```python
from build123d import *

# Parameters (mm, degrees)
F0_W     = 114
F0_H     = 114
F1_DEPTH = 50
F2_T     = -3
F4_DEPTH = 114.001
F6_DEPTH = 114.001
F7_R     = 5
F8_R     = 2
F9_R     = 2


with BuildPart() as f1:
    # F0 (on Top) → F1 (new body)
    with BuildSketch(Plane.XY):
        with Locations((24.0205488801, 21.5819291472)):
            Rectangle(F0_W, F0_H)
    extrude(amount=F1_DEPTH)

    # F2
    f2_openings = [f1.faces().sort_by_distance(p)[0] for p in [
        (24.020549, 21.581929, 50),
    ]]
    offset(amount=F2_T, openings=f2_openings)

    # F3 (on face) → F4 (cut, through all)
    with BuildSketch(Plane(origin=(-32.9794511199, 0, 0), x_dir=(0, -1, 0), z_dir=(-1, 0, 0))):
        with BuildLine():
            Line((-12.5819291472, 19), (-12.5819291472, 50))
            Line((-12.5819291472, 50), (-30.5819291472, 50))
            Line((-30.5819291472, 50), (-30.5819291472, 19))
            ThreePointArc((-30.5819291472, 19), (-21.5819291472, 10), (-12.5819291472, 19))
        make_face()
    extrude(amount=-F4_DEPTH, mode=Mode.SUBTRACT)

    # F5 (on face) → F6 (cut, through all)
    with BuildSketch(Plane(origin=(0, 78.5819291472, 0), x_dir=(-1, 0, 0), z_dir=(0, 1, 0))):
        with BuildLine():
            Line((-33.0205488801, 50), (-33.0205488801, 19))
            ThreePointArc((-33.0205488801, 19), (-24.0205488801, 10), (-15.0205488801, 19))
            Line((-15.0205488801, 19), (-15.0205488801, 50))
            Line((-15.0205488801, 50), (-33.0205488801, 50))
        make_face()
    extrude(amount=-F6_DEPTH, mode=Mode.SUBTRACT)

    # F7
    f7_edges = [f1.edges().sort_by_distance(p)[0] for p in [
        (15.020549, 77.081929, 50),
        (15.020549, -33.918071, 50),
        (33.020549, 77.081929, 50),
        (33.020549, -33.918071, 50),
        (79.520549, 12.581929, 50),
        (-31.479451, 12.581929, 50),
        (79.520549, 30.581929, 50),
        (-31.479451, 30.581929, 50),
    ]]
    fillet(f7_edges, radius=F7_R)

    # F8
    f8_edges = [f1.edges().sort_by_distance(p)[0] for p in [
        (81.020549, -35.418071, 25),
        (-32.979451, -35.418071, 25),
        (-32.979451, 78.581929, 25),
        (81.020549, 78.581929, 25),
    ]]
    fillet(f8_edges, radius=F8_R)

    # F9
    f9_edges = [f1.edges().sort_by_distance(p)[0] for p in [
        (-29.979451, -32.418071, 26.5),
        (-29.979451, 75.581929, 26.5),
        (78.020549, 75.581929, 26.5),
        (78.020549, -32.418071, 26.5),
    ]]
    fillet(f9_edges, radius=F9_R)


solid = f1.part
```
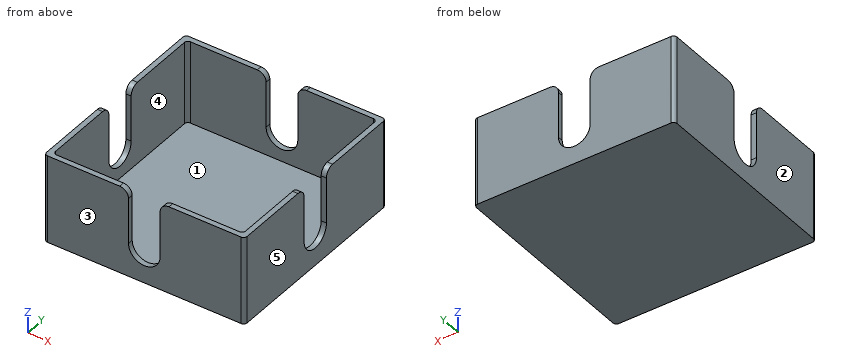
Geometry check sheet. Reference: the model listing, model coordinates, mm. Face numbers are marked on the shaded views. A direction names the side the tool comes from. Give positions to 0.01 mm unless a question says otherwise; leave off trailing zeros. Order: outer loops, then holes, each group sorted by start corner. A loop starts at its lowest first (then second) coordinate and runs counter-clockwise, first axis right, second up. Notation, with made-up numbers: (17.25, -21) - (32.25, -21) arc R16 cw to (32.25, -13) - close; hole circle Ø11 at (41.25, 68.5). An arc over 180 degrees is marked (long way). Answer in a Markdown table with one row per item. Add a question column.
Q1. Gauge pin test, flat ends, axial feed: pin 1 (8 mm diameter, centred on y = 20.5, z = 36.5, fed in from +X); pin 2 (2.5 mm diameter, centred on y = 77, z = 34.5, fed in from -X); pin 3 (4 mm diameter, centred on x = 69, y = 43, fed in from +Z). Record the tip position at first contact, or that the pin passes through.
Q2. Cross-section at C-C, the plane x = 63.5. Enter the section's corners in (y, z).
Q3. Material ranges on probe 1 along X at (y, z) = (-22, 3.5); probe 2 along Y at (x, z) = (-23, 19.5); probe 3 along Z at (x, y) = (7, 21.5), recorded low to high. Write a range as from..to.
Q4. Cross-section at B-B, the plane y = 40. Enter the section's corners in (x, z), then the cut area to 3 significant figures.
Q5. Tool access check on the marked faces 1 and 2. Record the directions out of +Z, -Z, +X, -X, +Y, -Y that give a thin tool (end or side, any length) a straight path to the whole face; none if there is none.
Q6. Cross-section at A-A, the plane z = 42. Count the separate pieces of the cut face and the enclosed holes in it, then the cut area to 3 significant figures.
Q7. Mould release check, pull along Y, two halves, no side actions. Record for the marked faces 3, 4 and 5: pulls with the +Y half, pulls with the -Y half, needs draft (parallel to the pull), parting line crosses it, or undercut.
Check values:
| question | item | result |
|---|---|---|
| 1 | pin 1 | passes through |
| 1 | pin 2 | stops at x = -32.98 |
| 1 | pin 3 | stops at z = 3 |
| 2 | outline | (-35.42, 0) - (78.58, 0) - (78.58, 50) - (75.58, 50) - (75.58, 3) - (-32.42, 3) - (-32.42, 50) - (-35.42, 50) - close |
| 3 | probe 1 | x = -32.98..-29.98, 78.02..81.02 |
| 3 | probe 2 | y = -35.42..-32.42, 75.58..78.58 |
| 3 | probe 3 | z = 0..3 |
| 4 | outline | (-32.98, 0) - (81.02, 0) - (81.02, 50) - (78.02, 50) - (78.02, 3) - (-29.98, 3) - (-29.98, 50) - (-32.98, 50) - close |
| 4 | area | 624 mm^2 |
| 5 | face 1 | +Z |
| 5 | face 2 | +Z, -Z, -X, +Y, -Y |
| 6 | separate pieces | 4 |
| 6 | enclosed holes | 0 |
| 6 | area | 1,120 mm^2 |
| 7 | face 3 | pulls with the -Y half |
| 7 | face 4 | undercut |
| 7 | face 5 | needs draft |
